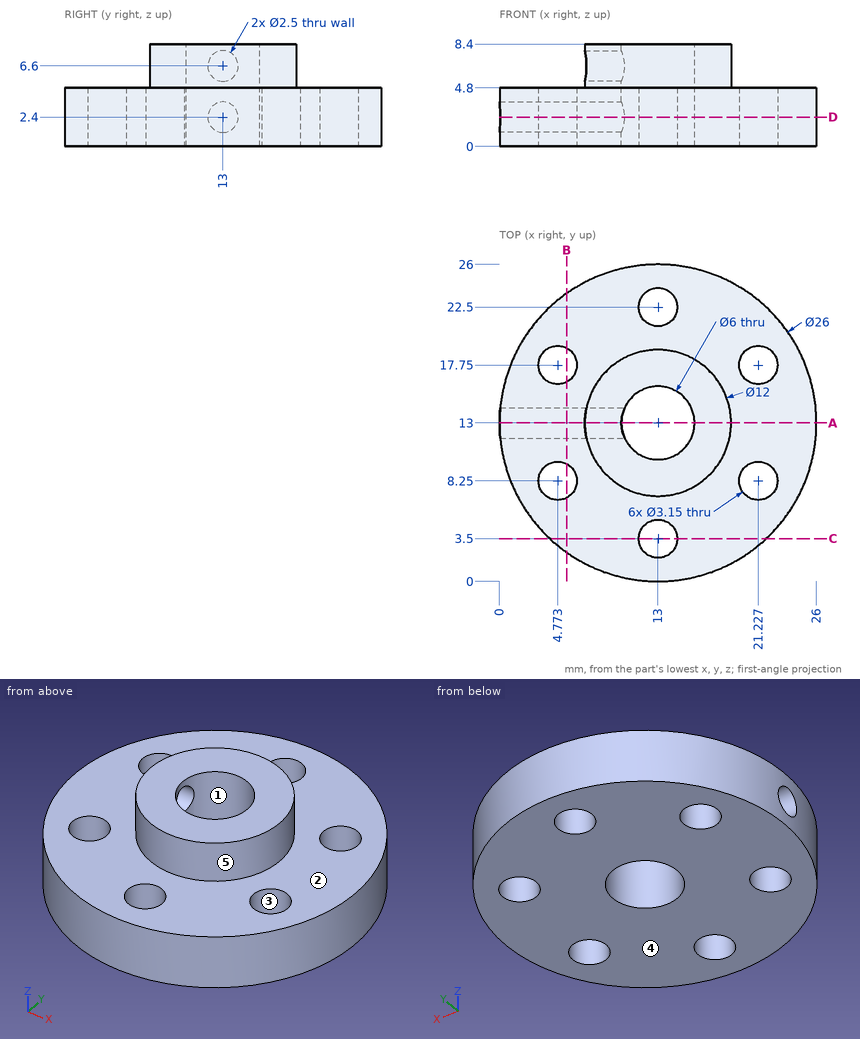
Job drawing, mm, ordinate dimensions from the low corner. One solid piece. A direction names the side the tool comes from. Give positions to 0.01 mm unless a question says otherwise; leave off trailing zeros. Order: outer loops, then holes, each group sorted by start corner. A loop starts at its lowest first (then second) coordinate and runs counter-clockwise, first axis right, second up. Notation, with made-up numbers: (62, 22.5) - (83, 22.5) arc R18 cw to (83, 43.5) - close; hole circle Ø8 at (25, 0). An arc over 180 degrees is marked (long way). Return JSON: item names as keys, results as strings.
1) Cut at B-B, the plane x = 5.5. Give the cut face in (y, z), plus the area to 3 significant figures.
Geometry says:
{"outline": "(2.38, 0) - (6.85, 0) - (6.85, 4.8) - (2.38, 4.8) - close; (9.65, 0) - (16.35, 0) - (16.35, 4.8) - (9.65, 4.8) - close; (19.15, 0) - (23.62, 0) - (23.62, 4.8) - (19.15, 4.8) - close; hole circle Ø2.5 at (13, 2.4)", "area": "70.2 mm²"}
2) Pull direction Y, two halves, no side cores. Call the marked faces 3, 4 and 5: pulls with the +Y half, pulls with the -Y half, needs draft (parallel to the pull), parting line crosses it, or undercut.
Geometry says:
{"face 3": "undercut", "face 4": "needs draft", "face 5": "parting line crosses it"}
3) Cut at D-D, the plane z = 2.4. Count the separate pieces of the cut face and the enclosed holes in it, plus the area to 3 significant figures.
Geometry says:
{"separate pieces": "1", "enclosed holes": "6", "area": "431 mm²"}
4) 3-axis set-ups, long thin cutter, end or side, ignore diameter. For the marked faces 1 and 2: which of +Z, -Z, +X, -X, +Y, -Y reach the whole face in a straight line?
Geometry says:
{"face 1": "+Z, -Z", "face 2": "+Z"}
5) Flat gauge pins, fed straight in: P1, Ø3.5, axis at x = 4.77, y = 17.75, coming from the +Z side; P2, Ø4, axis at y = 13, z = 3.5, coming from the -X side; P3, Ø3, axis at y = 13, z = 6.6, coming from the +X side; P4, Ø1, axis at x = 10, z = 4, coming from the -Y side. Where does each tip first touch, or does it go through?
Geometry says:
{"P1": "z = 4.8", "P2": "x = 0", "P3": "x = 19", "P4": "y = 0.24"}
6) Cut at A-A, the plane y = 13. Give the cut face in (x, z).
Geometry says:
{"outline": "(0, 0) - (10, 0) - (10, 1.15) - (0, 1.15) - close; (0, 3.65) - (10, 3.65) - (10, 5.35) - (7, 5.35) - (7, 4.8) - (0, 4.8) - close; (7, 7.85) - (10, 7.85) - (10, 8.4) - (7, 8.4) - close; (16, 0) - (26, 0) - (26, 4.8) - (19, 4.8) - (19, 8.4) - (16, 8.4) - close"}
7) Probe line 1 (X direction, y = 17.75, z = 2.95); line 2 (X direction, y = 8.75, z = 0.75) (1 decimal); line 3 (Z direction, x = 18.75, y = 17). List the from-to ranges inside material, lowest first. Write a range as from..to.
Geometry says:
{"line 1": "0.9..3.2, 6.35..19.65, 22.8..25.1", "line 2": "0.7..3.3, 6.3..19.7, 22.7..25.3", "line 3": "0..4.8"}
8) Cut at C-C, the plane y = 3.5. Give the cut face in (x, z) (1 decimal).
Geometry says:
{"outline": "(4.1, 0) - (11.4, 0) - (11.4, 4.8) - (4.1, 4.8) - close; (14.6, 0) - (21.9, 0) - (21.9, 4.8) - (14.6, 4.8) - close"}
